Design review of the part built by this model. Coordinates are the model's own, in mm. A direction names the side the tool comes from. Give positions to 0.01 mm unless a question says otherwise; leave off trailing zeros. Order: outer loops, then holes, each group sorted by start corner. A loop starts at its lowest first (then second) coordinate and runs counter-clockwise, first axis right, second up.
Autodesk Inventor part; units mm, degrees
ref_plane "YZ Plane" through (0, 0, 0) normal (1, 0, 0) x (0, 1, 0)
ref_plane "XZ Plane" through (0, 0, 0) normal (0, 1, 0) x (-1, 0, 0)
ref_plane "XY Plane" through (0, 0, 0) normal (0, 0, 1) x (1, 0, 0)
sketch "Sketch1" plane through (0, 0, 0) normal (0, 0, 1) x (1, 0, 0)
  line L0 (-20, 0) -> (20, 0)
  line L1 (20, 0) -> (20, -130)
  line L2 (20, -130) -> (-20, -130)
  line L3 (-20, -130) -> (-20, 0)
  point P0 (0, 0)
  point P1 (0, 0)
  dimension "d0" = 40
  dimension "d1" = 130
extrude "Plate1" add sketch "Sketch1" along normal blind 2
sketch "Sketch2" plane through (20, -130, 0) normal (1, 0, 0) x (0, 1, 0)
  line L0 (130, 0) -> (0, 0)
  line L1 (0, 0) -> (0, -33)
  line L2 (0, -33) -> (130, -33)
  line L3 (130, -33) -> (130, 0)
edge flange "Flange1" height 35 angle 90 thickness 2 bend radius 2.75 thickness toward (1, 0, 0) relief round relief width 2 relief depth 1 corner gap 2.75 corner form 0 edges at (20, -65, 0) (-20, -65, 0) wall of the first edge with corners at (20, 0, 0) (20, -130, 0) (20, -130, -33) (20, 0, -33)
bend "Bend1"
corner "Corner1"
sketch "Sketch3" plane through (0, 0, 0) normal (1, 0, 0) x (0, 1, 0)
  line L0 (0, -33) -> (-130, -33)
  line L1 (-115, -20) -> (-115, -20) construction
  line L2 (-117.5, -20) -> (-117.5, -20)
  line L3 (-112.5, -20) -> (-112.5, -20)
  arc A0 (-112.5, -20) -> (-117.5, -20) centre (-115, -20) ccw
  arc A1 (-117.5, -20) -> (-112.5, -20) centre (-115, -20) ccw
  line L4 (-130, -2.75) -> (-130, -33)
  point P0 (0, 0)
  point P1 (-115, -20)
  dimension "d14" = 0
  dimension "d15" = 13
  dimension "d17" = 2.5
  dimension "d18" = 15
extrude "Extrusion1" cut sketch "Sketch3" along normal through all both and the other way through all
sketch "Sketch6" plane through (0, 0, 2) normal (0, 0, 1) x (1, 0, 0)
  line L0 (-17.25, 0) -> (17.25, 0)
  circle A0 centre (0, -115) radius 2.5
  line L1 (22, -112.5) -> (22, -117.5)
  point P0 (0, 0)
  point P1 (0, 0)
  point P2 (22, -115)
  dimension "d27" = 5
extrude "Extrusion3" cut sketch "Sketch6" against normal blind 10
fillet "Fillet1" radius 2 4 edges at (21, 0, -33) (-21, 0, -33) (21, -130, -33) (-21, -130, -33)
pattern_linear "Rectangular Pattern2" count 2 spacing 100 along (0, 1, 0) of "Extrusion1", "Extrusion3"
equation "\"d2\" = Thickness"
equation "\"d3\" = BendReliefWidth"
equation "\"d4\" = BendReliefDepth"
equation "\"d5\" = MinimumRemnant"
equation "\"d6\" = TransitionRadius"
equation "\"d9\" = BendRadius"
equation "\"d10\" = CornerReliefSize"
equation "\"d11\" = GapSize"
equation "\"d12\" = JacobiRadiusSize"
equation "\"BendReliefWidth\" = Thickness"
equation "\"BendReliefDepth\" = 0.5 * Thickness"
equation "\"CornerReliefSize\" = 4 * Thickness"
equation "\"MinimumRemnant\" = 2 * Thickness"
equation "\"TransitionRadius\" = BendRadius"
equation "\"JacobiRadiusSize\" = BendRadius"
equation "\"GapSize\" = Thickness"
properties part number "NDM 11.027 bracket 27" material "Stainless Steel"
1. Take a section at B-B (y = -115). State the section outline as (x, z) points.
Recorded:
outline: (-22, -33) - (-20, -33) - (-20, -22.5) - (-22, -22.5) - close; (-22, -17.5) - (-20, -17.5) - (-20, -2.75) arc R2.75 cw to (-17.25, 0) - (-2.5, 0) - (-2.5, 2) - (-17.25, 2) arc R4.75 ccw to (-22, -2.75) - close; (2.5, 0) - (17.25, 0) arc R2.75 cw to (20, -2.75) - (20, -17.5) - (22, -17.5) - (22, -2.75) arc R4.75 ccw to (17.25, 2) - (2.5, 2) - close; (20, -33) - (22, -33) - (22, -22.5) - (20, -22.5) - close
2. Machinability: for faces 1 (the face through (20, -66, -18)), 2 (the face through (0, -130, 1)), which of the approach directions +Z, -Z, +X, -X, +Y, -Y give a long, thin tool a straight path to every point of the face, cutting with its end or side? Answer none if there is none.
Recorded:
face 1: -Z, +Y, -Y
face 2: +Z, -Z, +X, -X, -Y
3. Take a section at C-C (z = -28). State the section outline as (x, y) points, then the cut area to 3 significant figures.
Recorded:
outline: (-22, -130) - (-20, -130) - (-20, 0) - (-22, 0) - close; (20, -130) - (22, -130) - (22, 0) - (20, 0) - close
area: 520 mm2
4. For pin 1 (8 mm diameter, centred on x = 0, y = -15, fed in from -Z); pin 2 (10 mm diameter, centred on x = 13, z = -5.5, fed in from +Y), all flat-tipped, find the tip position at first contact; note any pin that passes through.
Recorded:
pin 1: stops at z = 0
pin 2: passes through
5. For line 1 along Y through (x, z) = (0, 1.65); line 2 along X through (y, z) = (-73.5, -10); line 3 along Z through (x, y) = (-4.5, -51.5), list the stretches that pass through material, from the lowest coordinate up.
Recorded:
line 1: y = -130 to -117.5, -112.5 to -17.5, -12.5 to 0
line 2: x = -22 to -20, 20 to 22
line 3: z = 0 to 2
6. Take a section at A-A (z = -20). State the section outline as (x, y) points, then the cut area to 3 significant figures.
Recorded:
outline: (-22, -130) - (-20, -130) - (-20, -117.5) - (-22, -117.5) - close; (-22, -112.5) - (-20, -112.5) - (-20, -17.5) - (-22, -17.5) - close; (-22, -12.5) - (-20, -12.5) - (-20, 0) - (-22, 0) - close; (20, -130) - (22, -130) - (22, -117.5) - (20, -117.5) - close; (20, -112.5) - (22, -112.5) - (22, -17.5) - (20, -17.5) - close; (20, -12.5) - (22, -12.5) - (22, 0) - (20, 0) - close
area: 480 mm2
7. Take a section at D-D (y = -87). State the section outline as (x, z) points, then the cut area to 3 significant figures.
Recorded:
outline: (-22, -33) - (-20, -33) - (-20, -2.75) arc R2.75 cw to (-17.25, 0) - (17.25, 0) arc R2.75 cw to (20, -2.75) - (20, -33) - (22, -33) - (22, -2.75) arc R4.75 ccw to (17.25, 2) - (-17.25, 2) arc R4.75 ccw to (-22, -2.75) - close
area: 214 mm2
8. Draft analysis for pull direction Z (two halves, no side actions). For faces 3 (the face through (-21.014, -117.385, -19.249)), 4 (the face through (-0.54, -17.44, 1.01)), 5 (the face through (-20.645, -64.09, 0.572)), 6 (the face through (-21, -12.5, -19.9)), state which applies: pulls with the +Z half, pulls with the -Z half, needs draft (parallel to the pull), parting line crosses it, or undercut.
Recorded:
face 3: undercut
face 4: needs draft
face 5: pulls with the +Z half
face 6: undercut
